CAD build for the part. Positions are in the model's coordinates, mm. Face numbers are marked on the shaded views. Round coordinates to 2 decimals unless told otherwise and drop trailing zeros. Loops run counter-clockwise (first coordinate to the right, second up) from the corner with the lowest first, then second, coordinate; pieces in that order, holes last. Notation, with made-up numbers: (-12.75, 24.5) - (1.25, 24.5) arc R34 cw to (1.25, 63.5) - close; hole circle Ø7 at (-1.75, 59). An arc over 180 degrees is marked (long way). One line per question, with ' | ' between items.
```python
from build123d import *

# Parameters (mm, degrees)
SKETCH1_R           = 50
SKETCH1_R_2         = 29
BOSS_EXTRUDE1_DEPTH = 4.5
SKETCH2_R           = 2.25
CUT_EXTRUDE1_DEPTH  = 10
CIRPATTERN1_COUNT   = 8


with BuildPart() as part:
    # Sketch1 → Boss-Extrude1 (new body, symmetric)
    with BuildSketch(Plane(origin=(0, 0, 0), x_dir=(1, 0, 0), z_dir=(0, 1, 0))):
        Circle(SKETCH1_R)
        Circle(SKETCH1_R_2, mode=Mode.SUBTRACT)
    extrude(amount=BOSS_EXTRUDE1_DEPTH, both=True)

    # Sketch2 → Cut-Extrude1 (cut, through all)
    with BuildSketch(Plane(origin=(0, 4.5, 0), x_dir=(1, 0, 0), z_dir=(0, 1, 0))):
        with Locations((0, 45.5)):
            Circle(SKETCH2_R)
    cut_extrude1 = extrude(amount=-CUT_EXTRUDE1_DEPTH, mode=Mode.SUBTRACT)

    # CirPattern1: Cut-Extrude1 ×8 about axis
    cirpattern1_axis = Axis((0, 0, 0), (0, 1, 0))
    for i in range(1, CIRPATTERN1_COUNT):
        add(cut_extrude1.rotate(cirpattern1_axis, i * 360 / CIRPATTERN1_COUNT), mode=Mode.SUBTRACT)


solid = part.part
```
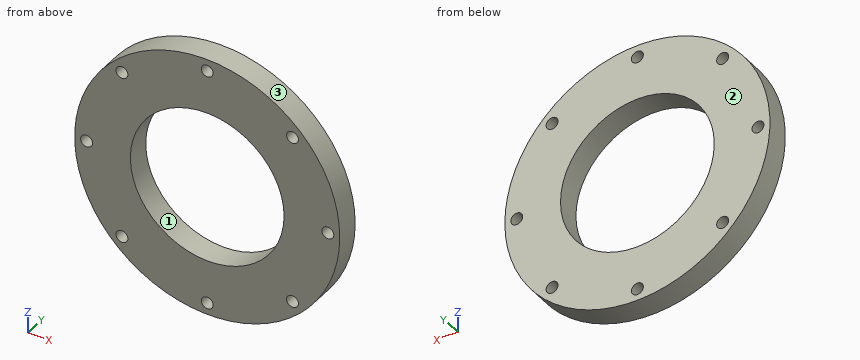
(1) Two-plate mould, pull along X, no slides. Class the marked faces 1, 2 and 3: released by +X, released by -X, zero draft, split by the parting line, or undercut.
Results found:
face 1: undercut | face 2: zero draft | face 3: split by the parting line
(2) Cut at C-C, the plane x = 27.5. Write the cut outline in (y, z).
Results found:
outline: (-4.5, -41.76) - (4.5, -41.76) - (4.5, -9.21) - (-4.5, -9.21) - close; (-4.5, 9.21) - (4.5, 9.21) - (4.5, 41.76) - (-4.5, 41.76) - close
(3) Cut at B-B, the plane x = 0. Write the cut outline in (y, z).
Results found:
outline: (-4.5, -50) - (4.5, -50) - (4.5, -47.75) - (-4.5, -47.75) - close; (-4.5, -43.25) - (4.5, -43.25) - (4.5, -29) - (-4.5, -29) - close; (-4.5, 29) - (4.5, 29) - (4.5, 43.25) - (-4.5, 43.25) - close; (-4.5, 47.75) - (4.5, 47.75) - (4.5, 50) - (-4.5, 50) - close
(4) Cut at D-D, the plane y = 0.25. State how many separate pieces and enclosed holes the cut face has, then the cut area to 3 significant figures.
Results found:
separate pieces: 1 | enclosed holes: 9 | area: 5,080 mm²
(5) Drop flat-ended pins along their axis: P1, Ø3.5, axis at x = 32.17, z = -32.17, coming from the +Y side; P2, Ø7, axis at x = 0, z = 45.5, coming from the +Y side; P3, Ø1, axis at y = 1.5, z = -25.5, coming from the -X side; P4, Ø4, axis at y = -3.5, z = 23.5, coming from the +X side. Give the stop position or say it passes through.
Results found:
P1: passes through | P2: stops at y = 4.5 | P3: stops at x = -43.3 | P4: stops at x = 45.14
(6) Cut at A-A, the plane z = 0. Write the cut outline in (x, y).
Results found:
outline: (-50, -4.5) - (-47.75, -4.5) - (-47.75, 4.5) - (-50, 4.5) - close; (-43.25, -4.5) - (-29, -4.5) - (-29, 4.5) - (-43.25, 4.5) - close; (29, -4.5) - (43.25, -4.5) - (43.25, 4.5) - (29, 4.5) - close; (47.75, -4.5) - (50, -4.5) - (50, 4.5) - (47.75, 4.5) - close
(7) Probe L1, parallel to X at y = 2.5, z = 0.5; L2, parallel to X at y = 1, z = -45.5; L3, parallel to X at y = -1, z = 24.5. List the from-to ranges inside material, lowest first.
Results found:
L1: x = -50 to -47.69, -43.31 to -29, 29 to 43.31, 47.69 to 50 | L2: x = -20.73 to -2.25, 2.25 to 20.73 | L3: x = -43.59 to -15.52, 15.52 to 43.59
